Source: CAD feature listing. Evaluate the final solid. Frame: model axes, mm. Face numbers are marked on the shaded views. Round coordinates to 2 decimals unless told otherwise and drop trailing zeros. Order: outer loops, then holes, each group sorted by start corner. A loop starts at its lowest first (then second) coordinate and runs counter-clockwise, first axis right, second up. Notation, with made-up numbers: (38.25, 41.5) - (48.25, 41.5) arc R25 cw to (48.25, 76.5) - close; hole circle Ø10 at (-14, 83.25). An arc over 180 degrees is marked (long way). Use one line per item in the form item = value. Start each with the question number.
Q1. Draft query along Y for the marked faces 1 and 2. Return one class per face: released by +Y, released by -Y, zero draft, split by the parting line, or undercut.
Q2. Cut plane C-C, the plane x = 26.5. Return the cut outline in (y, z) (3 decimals).
Q3. Cut plane B-B, the plane y = 2. Return the cut outline in (x, z), and give its area (3 significant figures).
Q4. Pin query (flat end, axial travel): pin 1 Ø3 at (x, y) = (106, 14) entering from +Z; pin 2 Ø8 at (x, z) = (16.5, -0.5) entering from -Y (3 decimals); pin 3 Ø3 at (x, z) = (107, -0.5) entering from +Y; pin 4 Ø2.5 at (x, y) = (95, 14.5) entering from -Z. Return the tip coordinate at first contact, or that it passes through.
Q5. Cut plane D-D, the plane z = -6. Return the cut outline in (x, y), and give its area (3 significant figures).
Q6. Cut plane A-A, the plane z = 0. Return the cut outline in (x, y) (1 decimal).
Q7. Ray query, line 1 (X direction, y = -11, z = 7); line 2 (Z direction, x = 6.5, y = -2); line 3 (Z direction, x = 38, y = 9). Return the intervals inside material, ascending. Write a range as [from, to].
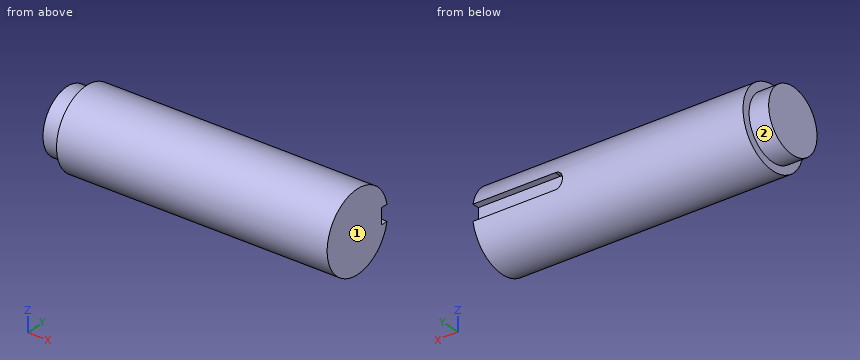
Autodesk Inventor part; units mm, degrees
ref_plane "YZ Plane" through (0, 0, 0) normal (1, 0, 0) x (0, 1, 0)
ref_plane "XZ Plane" through (0, 0, 0) normal (0, 1, 0) x (-1, 0, 0)
ref_plane "XY Plane" through (0, 0, 0) normal (0, 0, 1) x (1, 0, 0)
sketch "Sketch1" plane through (0, 0, 0) normal (1, 0, 0) x (0, 1, 0)
  circle A0 centre (0, 0) radius 15.875
  dimension "d0" = 31.75
extrude "Extrusion1" add sketch "Sketch1" along normal blind 117.7036
ref_plane "Work Plane1" through (65.5447, 0, 0) normal (1, 0, 0) x (0, 0, -1)
sketch "Sketch9" plane through (117.7036, 0, 0) normal (1, 0, 0) x (0, 0, -1)
  line L0 (-3.175, 15.875) -> (-3.175, 12.7)
  line L1 (-3.175, 12.7) -> (3.175, 12.7)
  line L2 (3.175, 12.7) -> (3.175, 15.875)
  line L3 (0, 0) -> (0, 19.977)
  circle A0 centre (0, 0) radius 15.875
  line L4 (0, 15.875) -> (-16.159, 15.875)
  point P0 (0, 12.7)
  point P1 (3.175, 15.5543)
  point P2 (-3.175, 15.5543)
  dimension "d26" = 6.35
  dimension "d27" = 3.175
extrude "Extrusion9" cut sketch "Sketch9" against normal blind 33.3502 contours A0 L3 L1 L0 | A0 L2 L1 L3
sketch "Sketch10" plane through (0, 0, 0) normal (-1, 0, 0) x (0, 0, 1)
  circle A0 centre (0, 0) radius 15.875
  circle A1 centre (0, 0) radius 12.7
  dimension "d30" = 25.4
extrude "Extrusion10" cut sketch "Sketch10" against normal blind 7.9375
sketch "Sketch11" plane through (117.7036, 12.7, 3.175) normal (0, 1, 0) x (1, 0, 0)
  line L0 (0, 0) -> (-33.3502, 0)
  line L1 (-33.3502, 6.35) -> (0, 6.35)
  line L2 (-33.3502, 6.35) -> (-33.3502, 0)
  arc A0 (-36.4412, 5.0705) -> (-33.3502, 0) centre (-39.0546, 0) ccw
  circle A1 centre (-33.3502, 3.175) radius 3.175
  point P0 (-117.7036, 3.175)
extrude "Extrusion11" cut sketch "Sketch11" along normal blind 25.4
properties part number "DTR-3"
Completed:
q1.face_1 = zero draft
q1.face_2 = split by the parting line
q2.outline = circle Ø31.75 at (0, 0)
q3.outline = (0, -12.54) - (7.94, -12.54) - (7.94, -15.75) - (117.7, -15.75) - (117.7, 15.75) - (7.94, 15.75) - (7.94, 12.54) - (0, 12.54) - close
q3.area = 3,660 mm2
q4.pin_1 = 9.79
q4.pin_2 = -15.875
q4.pin_3 = 12.7
q4.pin_4 = -8.74
q5.outline = (0, -11.19) - (7.94, -11.19) - (7.94, -14.7) - (117.7, -14.7) - (117.7, 14.7) - (7.94, 14.7) - (7.94, 11.19) - (0, 11.19) - close
q5.area = 3,400 mm2
q6.outline = (0, -12.7) - (7.9, -12.7) - (7.9, -15.9) - (117.7, -15.9) - (117.7, 12.7) - (81.2, 12.7) - (81.2, 15.9) - (7.9, 15.9) - (7.9, 12.7) - (0, 12.7) - close
q7.line_1 = [7.94, 117.7]
q7.line_2 = [-12.54, 12.54]
q7.line_3 = [-13.08, 13.08]
